from build123d import *

# Parameters (mm, degrees)
BOSS_EXTRUDE1_DEPTH = 25.4
SKETCH3_W           = 27.94
SKETCH3_H           = 13.830872484
CUT_EXTRUDE1_DEPTH  = 77.2
FILLET1_R           = 1.5875
SKETCH4_R           = 3.3782
CUT_EXTRUDE2_DEPTH  = 60.652834174
SKETCH5_R           = 2.000000064
SKETCH5_R_2         = 12.55
CUT_EXTRUDE3_DEPTH  = 62.224011629


with BuildPart() as part:
    # Sketch2 → Boss-Extrude1 (new, symmetric)
    with BuildSketch(Plane.XY):
        with BuildLine():
            Line((-25.4, 0), (25.4, 0))
            Line((25.4, 0), (25.4, 50.8))
            Line((25.4, 50.8), (23.8125, 50.8))
            ThreePointArc((23.8125, 50.8), (22.689967985, 50.335032015), (22.225, 49.2125))
            Line((22.225, 49.2125), (22.225, 9.525))
            ThreePointArc((22.225, 9.525), (20.365128061, 5.034871939), (15.875, 3.175))
            Line((15.875, 3.175), (-23.8125, 3.175))
            ThreePointArc((-23.8125, 3.175), (-24.935032015, 2.710032015), (-25.4, 1.5875))
            Line((-25.4, 1.5875), (-25.4, 0))
        make_face()
    extrude(amount=BOSS_EXTRUDE1_DEPTH, both=True)

    # Sketch3 → Cut-Extrude1 (cut, through all)
    with BuildSketch(Plane(origin=(0, 0, -25.4), x_dir=(-1, 0, 0), z_dir=(0, 0, -1))):
        with Locations((11.43, 1.484116331)):
            Rectangle(SKETCH3_W, SKETCH3_H)
    extrude(amount=-CUT_EXTRUDE1_DEPTH, mode=Mode.SUBTRACT)

    # Fillet1
    fillet1_edges = [part.edges().sort_by_distance(p)[0] for p in [
        (2.54, 3.175, 0),
    ]]
    fillet(fillet1_edges, radius=FILLET1_R)

    # Sketch4 → Cut-Extrude2 (cut, through all)
    with BuildSketch(Plane(origin=(0, 3.175, 0), x_dir=(1, 0, 0), z_dir=(0, 1, 0))):
        with Locations(Location((10.00125, 12.7, 0), (0, 0, 180))):
            Circle(SKETCH4_R)
        with Locations(Location((10.00125, -12.7, 0), (0, 0, 180))):
            Circle(SKETCH4_R)
    extrude(amount=-CUT_EXTRUDE2_DEPTH, mode=Mode.SUBTRACT)

    # Sketch5 → Cut-Extrude3 (cut, through all)
    with BuildSketch(Plane(origin=(25.4, 0, 0), x_dir=(0, 0, -1), z_dir=(1, 0, 0))):
        with Locations((12.72792202, 16.6)):
            Circle(SKETCH5_R)
        with Locations((-12.72792202, 16.6)):
            Circle(SKETCH5_R)
        with Locations((-12.72792202, 42.055844039)):
            Circle(SKETCH5_R)
        with Locations((12.72792202, 42.055844039)):
            Circle(SKETCH5_R)
        with Locations((0, 29.32792202)):
            Circle(SKETCH5_R_2)
    extrude(amount=-CUT_EXTRUDE3_DEPTH, mode=Mode.SUBTRACT)


solid = part.part
Read the model definition and answer for the solid it produces. Units are mm, in the model's axes. A direction names the side the tool comes from. Coordinates: 2 decimals unless noted, no trailing zeros. Loops run counter-clockwise (first coordinate to the right, second up) from the corner with the lowest first, then second, coordinate; pieces in that order, holes last. Notation, with made-up numbers: (61, -16) -> (119, -16) arc R21 ccw to (119, 17) -> close; hole circle Ø3 at (-22.5, 52.25). An arc over 180 degrees is marked (long way). Answer in a Markdown table with one row per item.
Item 1: A cutting plane is placed at B-B on x = 7.5. Determine the outline of the cut face in (y, z) (3 decimals).
Returned:
| item | result |
|---|---|
| outline | (0, -25.4) -> (3.175, -25.4) -> (3.175, -14.971) -> (0, -14.971) -> close; (0, -10.429) -> (3.175, -10.429) -> (3.175, 10.429) -> (0, 10.429) -> close; (0, 14.971) -> (3.175, 14.971) -> (3.175, 25.4) -> (0, 25.4) -> close |
Item 2: A cutting plane is placed at C-C on y = 23. Determine the outline of the cut face in (x, z) (3 decimals), plus the area to 3 significant figures.
Returned:
| item | result |
|---|---|
| outline | (22.225, -25.4) -> (25.4, -25.4) -> (25.4, -10.838) -> (22.225, -10.838) -> close; (22.225, 10.838) -> (25.4, 10.838) -> (25.4, 25.4) -> (22.225, 25.4) -> close |
| area | 92.5 mm^2 |
Item 3: Each of these flat-tipped pins is pushed along its axis until it touches: P1, Ø11, axis at x = 10, z = 12.7, coming from the +Y side (3 decimals); P2, Ø6.5, axis at y = 42.06, z = -12.73, coming from the +X side; P3, Ø1, axis at x = 18.5, z = -12.5, coming from the +Y side; P4, Ø1, axis at y = 43, z = -17, coming from the -X side (3 decimals). Where does it stop, or does it pass through?
Returned:
| item | result |
|---|---|
| P1 | stops at y = 3.175 |
| P2 | stops at x = 25.4 |
| P3 | stops at y = 4 |
| P4 | stops at x = 22.225 |
Item 4: For faces 4 (the flat face through (22.4, 18, 25.4)), 5 (the flat face through (10, 3.175, 0)), determine the directions among +Z, -Z, +X, -X, +Y, -Y from which every point of the face is accessible in a straight line to the end or side of a thin tool.
Returned:
| item | result |
|---|---|
| face 4 | +Z, +X, -X, +Y, -Y |
| face 5 | +Z, -Z, -X, +Y |
Item 5: Straight lines are drawn through the part: line 1 along Y through (x, z) = (12.75, 3) (3 decimals); line 2 along X through (y, z) = (1, 12); line 3 along X through (y, z) = (28, 19) (3 decimals). For each, find the intervals that lie inside material, in ascending order. Write a range as [from, to].
Returned:
| item | result |
|---|---|
| line 1 | y = [0, 3.175] |
| line 2 | x = [2.54, 6.7], [13.31, 25.4] |
| line 3 | x = [22.225, 25.4] |
Item 6: For a pull along Y with two mould halves and no side action, classify faces 1 (the cylindrical face through (23.835, 15.834, -14.575)), 2 (the cylindrical face through (22.702, 50.347, 0.356)), 3 (the flat face through (22.225, 34, 12)) as released by +Y, released by -Y, zero draft, split by the parting line, or undercut.
Returned:
| item | result |
|---|---|
| face 1 | undercut |
| face 2 | released by +Y |
| face 3 | zero draft |
